For this review, take the finished solid that the model builds, in its own axes (mm). Face numbers are marked on the shaded views. Round coordinates to 2 decimals unless told otherwise and drop trailing zeros. Order: outer loops, then holes, each group sorted by start corner. A loop starts at its lowest first (then second) coordinate and runs counter-clockwise, first axis right, second up. Notation, with made-up numbers: (-3.75, 22.5) -> (11.25, 22.5) arc R22 ccw to (11.25, 57.5) -> close; hole circle Ø11 at (79, 61.25). An arc over 180 degrees is marked (long way). Answer in a Markdown table with one row per item.
```python
from build123d import *

# Parameters (mm, degrees)
F0_R     = 1.25
F0_R_2   = 0.75
F0_R_3   = 4.25
F1_DEPTH = 3.175


# Not quite as in the source:
# - a length typed as a fraction of an inch, garbled in the dataset ("3 / 203.2 mm" for 3/8 in), is restored


with BuildPart() as f1:
    # F0 (on Top) → F1 (new body)
    with BuildSketch(Plane.XY):
        with BuildLine():
            Line((-38.4956756474, 4.4767191038), (-32.8665105228, 14.2267191038))
            ThreePointArc((-32.8665105228, 14.2267191038), (-41.3102582097, 28.8517191038), (-49.7540058966, 14.2267191038))
            Line((-49.7540058966, 14.2267191038), (-44.124840772, 4.4767191038))
            ThreePointArc((-44.124840772, 4.4767191038), (-41.3102582097, 2.8517191038), (-38.4956756474, 4.4767191038))
        make_face()
        with Locations((-41.3102582097, 6.1017191038)):
            Circle(F0_R, mode=Mode.SUBTRACT)
        with Locations((-41.3102582097, 12.1017191038)):
            Circle(F0_R_2, mode=Mode.SUBTRACT)
        with Locations((-48.3102582097, 19.1017191038)):
            Circle(F0_R_2, mode=Mode.SUBTRACT)
        with Locations((-41.3102582097, 19.1017191038)):
            Circle(F0_R_3, mode=Mode.SUBTRACT)
        with Locations((-34.3102582097, 19.1017191038)):
            Circle(F0_R_2, mode=Mode.SUBTRACT)
        with Locations((-41.3102582097, 26.1017191038)):
            Circle(F0_R_2, mode=Mode.SUBTRACT)
    extrude(amount=F1_DEPTH)


solid = f1.part
```
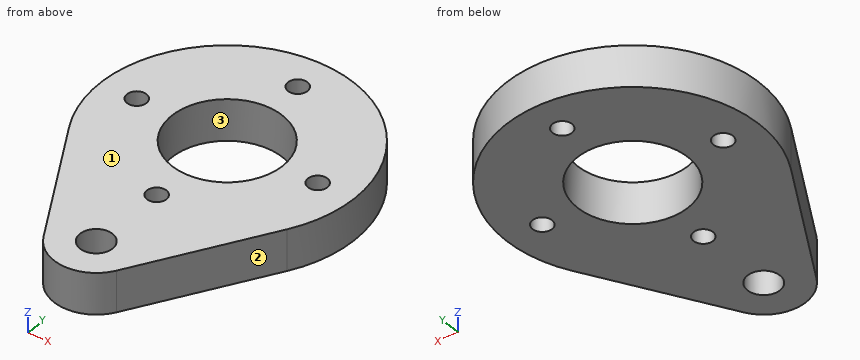
Q1. Take a section at C-C, the plane y = 18.75. Write out the cut boundary in (x, z) (3 decimals), then the cut area to 3 significant figures.
Answer key:
| item | result |
|---|---|
| outline | (-51.054, 0) -> (-48.973, 0) -> (-48.973, 3.175) -> (-51.054, 3.175) -> close; (-47.648, 0) -> (-45.546, 0) -> (-45.546, 3.175) -> (-47.648, 3.175) -> close; (-37.075, 0) -> (-34.973, 0) -> (-34.973, 3.175) -> (-37.075, 3.175) -> close; (-33.648, 0) -> (-31.567, 0) -> (-31.567, 3.175) -> (-33.648, 3.175) -> close |
| area | 26.6 mm^2 |
Q2. Take a section at D-D, the plane z = 1.85. Write out the cut boundary in (x, y), then the cut area to 3 significant figures.
Answer key:
| item | result |
|---|---|
| outline | (-49.75, 14.23) -> (-44.12, 4.48) arc R3.25 ccw to (-38.5, 4.48) -> (-32.87, 14.23) arc R9.75 ccw (long way) to start; hole circle Ø1.5 at (-48.31, 19.1); hole circle Ø8.5 at (-41.31, 19.1); hole circle Ø2.5 at (-41.31, 6.1); hole circle Ø1.5 at (-41.31, 12.1); hole circle Ø1.5 at (-41.31, 26.1); hole circle Ø1.5 at (-34.31, 19.1) |
| area | 288 mm^2 |
Q3. Clearance check with a flat-ended pin moving along its axis: pin 1 Ø1 at (x, z) = (-34.5, 0.5) entering from -Y. State where the tip first meets the part, or that it passes through.
Answer key:
| item | result |
|---|---|
| pin 1 | stops at y = 10.53 |
Q4. To check wall thickness, follow probe 1 along Y at (x, z) = (-41.5, 1.6); probe 2 along X at (y, z) = (18.5, 1.45); probe 3 along X at (y, z) = (6, 2.4). State the ranges of each line that lie inside material, in increasing order.
Answer key:
| item | result |
|---|---|
| probe 1 | y = 2.86 to 4.87, 7.34 to 11.38, 12.83 to 14.86, 23.35 to 25.38, 26.83 to 28.85 |
| probe 2 | x = -51.04 to -48.76, -47.86 to -45.52, -37.1 to -34.76, -33.86 to -31.58 |
| probe 3 | x = -45 to -42.56, -40.06 to -37.62 |
Q5. The part is to be moulded in two halves that separate along X. For the marked faces 1, 2 and 3, say which applies: +X half, -X half, draft (parallel to the pull), parting line (faces both ways), or undercut.
Answer key:
| item | result |
|---|---|
| face 1 | draft |
| face 2 | +X half |
| face 3 | undercut |
Q6. Take a section at B-B, the plane x = -45. Write out the cut boundary in (y, z) (3 decimals), then the cut area to 3 significant figures.
Answer key:
| item | result |
|---|---|
| outline | (5.993, 0) -> (16.993, 0) -> (16.993, 3.175) -> (5.993, 3.175) -> close; (21.211, 0) -> (28.127, 0) -> (28.127, 3.175) -> (21.211, 3.175) -> close |
| area | 56.9 mm^2 |
Q7. Take a section at A-A, the plane y = 21.5. Write out the cut boundary in (x, z) (3 decimals).
Answer key:
| item | result |
|---|---|
| outline | (-50.761, 0) -> (-44.819, 0) -> (-44.819, 3.175) -> (-50.761, 3.175) -> close; (-37.802, 0) -> (-31.86, 0) -> (-31.86, 3.175) -> (-37.802, 3.175) -> close |
